```python
from build123d import *

# Parameters (mm, degrees)
F0_R     = 31.5
F1_DEPTH = 1
F2_R     = 5.25
F3_DEPTH = 1
F4_R     = 1.5
F4_R_2   = 2.35
F5_DEPTH = 1


with BuildPart() as f1:
    # F0 (on Top) → F1 (new body)
    with BuildSketch(Plane.XY):
        Circle(F0_R)
    extrude(amount=F1_DEPTH)

    # F2 (on face) → F3 (cut, through all)
    with BuildSketch(Plane.XY.offset(1)):
        Circle(F2_R)
    extrude(amount=-F3_DEPTH, mode=Mode.SUBTRACT)

    # F4 (on face) → F5 (cut, through all)
    with BuildSketch(Plane.XY.offset(1)):
        with BuildLine():
            Line((-5, 5.59017), (-5, 24.494897))
            ThreePointArc((-5, 24.494897), (-17.67767, 17.67767), (-24.494897, 5))
            Line((-24.494897, 5), (-5.59017, 5))
            ThreePointArc((-5.59017, 5), (-5.303301, 5.303301), (-5, 5.59017))
        make_face()
        with BuildLine():
            Line((5.59017, 5), (24.494897, 5))
            ThreePointArc((24.494897, 5), (17.67767, 17.67767), (5, 24.494897))
            Line((5, 24.494897), (5, 5.59017))
            ThreePointArc((5, 5.59017), (5.303301, 5.303301), (5.59017, 5))
        make_face()
        with BuildLine():
            ThreePointArc((5, -24.494897), (17.67767, -17.67767), (24.494897, -5))
            Line((24.494897, -5), (5.59017, -5))
            ThreePointArc((5.59017, -5), (5.303301, -5.303301), (5, -5.59017))
            Line((5, -5.59017), (5, -24.494897))
        make_face()
        with BuildLine():
            ThreePointArc((-24.494897, -5), (-17.67767, -17.67767), (-5, -24.494897))
            Line((-5, -24.494897), (-5, -5.59017))
            ThreePointArc((-5, -5.59017), (-5.303301, -5.303301), (-5.59017, -5))
            Line((-5.59017, -5), (-24.494897, -5))
        make_face()
        with Locations((0, -12)):
            Circle(F4_R)
        with Locations((15.5, 0)):
            Circle(F4_R_2)
        with Locations((0, 12)):
            Circle(F4_R)
        with Locations((-15.5, 0)):
            Circle(F4_R_2)
    extrude(amount=-F5_DEPTH, mode=Mode.SUBTRACT)


solid = f1.part
```
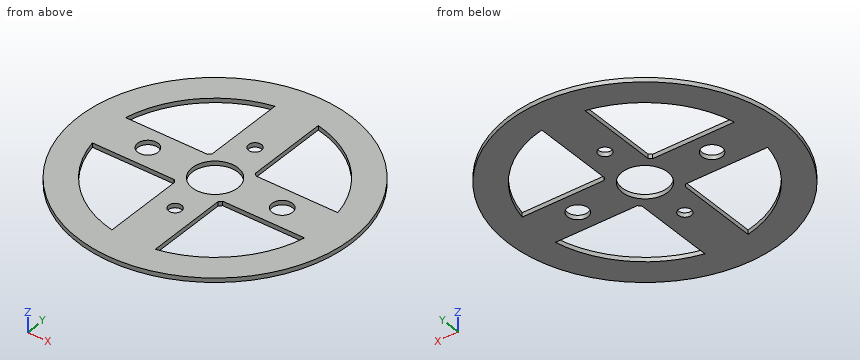
Input: part model. Units: mm. Frame: model coordinates. Round coordinates to 2 decimals unless told otherwise and drop trailing zeros. Order: outer loops, then holes, each group sorted by start corner. A loop starts at its lowest first (then second) coordinate and runs counter-clockwise, first axis right, second up. Notation, with made-up numbers: (66, -28.5) - (98, -28.5) arc R14 ccw to (98, -12.5) - close; hole circle Ø7 at (-29.75, -16). An arc over 180 degrees is marked (long way). One line per question, with ' | ' between items. Start each with the question number.
1) Contact query for flat-ended pins moving along their axis: P1, Ø8, axis at x = -13.5, y = -10, coming from the +Z side; P2, Ø0.5, axis at y = -18, z = 0.5, coming from the -X side. Output: stop coordinate, or through.
2) Cut plane B-B, the plane y = -12. Return the cut outline in (x, z), then the cut area to 3 significant figures.
3) Cut plane A-A, the plane z = 0.8. Give the number of separate pieces and of enclosed holes in the cut face, then the cut area to 3 significant figures.
4) Cut plane D-D, the plane x = 22. Return the cut outline in (y, z).
5) Cut plane C-C, the plane x = 0. Return the cut outline in (y, z).
6) Ray query, probe 1 along Y at (x, z) = (0, 0.2); probe 2 along X at (y, z) = (-1, 0.3); probe 3 along Y at (x, z) = (11.5, 0.25). Return the intervals inside material, ascending.
Worked out:
1) P1: passes through | P2: stops at x = -26.02
2) outline: (-29.12, 0) - (-21.93, 0) - (-21.93, 1) - (-29.12, 1) - close; (-5, 0) - (-1.5, 0) - (-1.5, 1) - (-5, 1) - close; (1.5, 0) - (5, 0) - (5, 1) - (1.5, 1) - close; (21.93, 0) - (29.12, 0) - (29.12, 1) - (21.93, 1) - close | area: 21.4 mm^2
3) separate pieces: 1 | enclosed holes: 9 | area: 1,910 mm^2
4) outline: (-22.54, 0) - (-11.87, 0) - (-11.87, 1) - (-22.54, 1) - close; (-5, 0) - (5, 0) - (5, 1) - (-5, 1) - close; (11.87, 0) - (22.54, 0) - (22.54, 1) - (11.87, 1) - close
5) outline: (-31.5, 0) - (-13.5, 0) - (-13.5, 1) - (-31.5, 1) - close; (-10.5, 0) - (-5.25, 0) - (-5.25, 1) - (-10.5, 1) - close; (5.25, 0) - (10.5, 0) - (10.5, 1) - (5.25, 1) - close; (13.5, 0) - (31.5, 0) - (31.5, 1) - (13.5, 1) - close
6) probe 1: y = -31.5 to -13.5, -10.5 to -5.25, 5.25 to 10.5, 13.5 to 31.5 | probe 2: x = -31.48 to -17.63, -13.37 to -5.15, 5.15 to 13.37, 17.63 to 31.48 | probe 3: y = -29.33 to -22.2, -5 to 5, 22.2 to 29.33
